Input: part model. Units: mm. Frame: model coordinates. A direction names the side the tool comes from. Coordinates: 2 decimals unless noted, no trailing zeros. Write each loop counter-clockwise with the first axis right and the second up, starting at its lowest first coordinate (ties: lowest second). Pieces come first, ordered by that corner, then holes. Notation, with made-up numbers: (-10, 7.5) - (1, 7.5) arc R13 ccw to (1, 23.5) - close; hole circle Ø2 at (-2, 60). An arc over 180 degrees is marked (long way). Use a Markdown table: item, result. Add a question column.
Q1. Pin query (flat end, axial travel): P1, Ø10, axis at x = -28.5, y = -15, coming from the -Z side; P2, Ø4, axis at x = -10.49, y = -152.4, coming from the -Z side; P3, Ø1.5, axis at x = -28.5, y = 143.5, coming from the -Z side; P4, Ø8.5, axis at y = -76.2, z = 228.6, coming from the +X side. Return the tip coordinate at first contact, or that it passes through.
Q2. Set-up query: faces 1 (the face through (1.6, 3, 3)), 2 (the face through (-36, -3, -217.5)), 3 (the face through (-35, -3, -215.9)), 4 (the face through (-12, -3, 242.9)), 5 (the face through (-23.8, -3, 226)). Return all of +Z, -Z, +X, -X, +Y, -Y with unobstructed straight access to the full face (end or side cutting, diameter ignored); none if empty.
Q3. Section query A-A (y = -59). Return the cut outline in (x, z).
Q4. Mould query, pull axis Z, two halves, no side actions, for faces 6 (the face through (1, -190.5, -73)), 7 (the face through (-23.513, 3, -229)), 8 (the face through (-12, -3, 241.3)), 9 (the face through (-14, 3, -242.9)). Classes: released by +Z, released by -Z, zero draft, split by the parting line, or undercut.
Q5. Section query B-B (z = -13). Return the cut outline in (x, y), then the cut area to 3 significant figures.
Q6. Material intervals for probe 1 along Y at (x, z) = (-24, 228); probe 2 along Z at (x, y) = (-7.5, 20); probe 3 along Y at (x, z) = (0.8, 228.6), sorted ascending. Write a range as from..to.
from build123d import *

# Parameters (mm, degrees)
SKETCH1_W                    = 482.6
SKETCH1_H                    = 381
BOSS_EXTRUDE1_DEPTH          = 1.6002
EDGE_FLANGE1_STRIP_W         = 9.6012
EDGE_FLANGE1_STRIP_H         = 1.6002
EDGE_FLANGE1_STRIP_CUT_DEPTH = 381
EDGE_FLANGE1_DEPTH           = 381
EDGE_FLANGE2_STRIP_W         = 9.6012
EDGE_FLANGE2_STRIP_H         = 1.6002
EDGE_FLANGE2_STRIP_CUT_DEPTH = 381
EDGE_FLANGE2_DEPTH           = 381
EDGE_FLANGE3_STRIP_W         = 9.6012
EDGE_FLANGE3_STRIP_H         = 1.6002
EDGE_FLANGE3_STRIP_CUT_DEPTH = 381
EDGE_FLANGE3_DEPTH           = 381
EDGE_FLANGE4_STRIP_W         = 9.6012
EDGE_FLANGE4_STRIP_H         = 1.6002
EDGE_FLANGE4_STRIP_CUT_DEPTH = 381
EDGE_FLANGE4_DEPTH           = 381
EDGE_FLANGE5_STRIP_W         = 9.6012
EDGE_FLANGE5_STRIP_H         = 1.6002
EDGE_FLANGE5_STRIP_CUT_DEPTH = 381
EDGE_FLANGE5_DEPTH           = 381
SKETCH24_R                   = 3.2639
CUT_EXTRUDE2_DEPTH           = 2.54
SKETCH25_R                   = 3.2639
CUT_EXTRUDE3_DEPTH           = 310.870566463
SKETCH26_R                   = 3.2639
CUT_EXTRUDE4_DEPTH           = 2.54
SKETCH27_R                   = 3.2639
CUT_EXTRUDE6_DEPTH           = 2.54
SKETCH29_R                   = 3.2639
CUT_EXTRUDE7_DEPTH           = 2.54


# Sheet-metal steps are written as plain solids
with BuildPart() as part:
    # Sketch1 → Boss-Extrude1 (new body)
    with BuildSketch(Plane(origin=(0, 0, 0), x_dir=(0, 0, -1), z_dir=(1, 0, 0))):
        Rectangle(SKETCH1_W, SKETCH1_H)
    extrude(amount=BOSS_EXTRUDE1_DEPTH)

    # Edge-Flange1 strip (across the edge) → Edge-Flange1 strip cut (cut)
    with BuildSketch(Plane(origin=(0, 190.5, -241.3), x_dir=(0, 0, 1), z_dir=(0, -1, 0))):
        with Locations((-3.2004, -0.8001)):
            Rectangle(EDGE_FLANGE1_STRIP_W, EDGE_FLANGE1_STRIP_H)
    extrude(amount=EDGE_FLANGE1_STRIP_CUT_DEPTH, mode=Mode.SUBTRACT)

    # Edge-Flange1 section (across the edge) → Edge-Flange1 (add)
    with BuildSketch(Plane(origin=(0, 190.5, -241.3), x_dir=(0, 0, 1), z_dir=(0, -1, 0))):
        with BuildLine():
            Line((-1.6002, 1.6002), (-1.6002, 23.51278))
            Line((-1.6002, 23.51278), (0, 23.51278))
            Line((0, 23.51278), (0, 1.6002))
            ThreePointArc((0, 1.6002), (0.468687729, 0.468687729), (1.6002, 0))
            Line((1.6002, 0), (1.6002, -1.6002))
            ThreePointArc((1.6002, -1.6002), (-0.662824543, -0.662824543), (-1.6002, 1.6002))
        make_face()
    extrude(amount=EDGE_FLANGE1_DEPTH)

    # Edge-Flange2 strip (across the edge) → Edge-Flange2 strip cut (cut)
    with BuildSketch(Plane(origin=(-23.51278, 190.5, -241.3), x_dir=(1, 0, 0), z_dir=(0, -1, 0))):
        with Locations((-3.2004, -0.8001)):
            Rectangle(EDGE_FLANGE2_STRIP_W, EDGE_FLANGE2_STRIP_H)
    extrude(amount=EDGE_FLANGE2_STRIP_CUT_DEPTH, mode=Mode.SUBTRACT)

    # Edge-Flange2 section (across the edge) → Edge-Flange2 (add)
    with BuildSketch(Plane(origin=(-23.51278, 190.5, -241.3), x_dir=(1, 0, 0), z_dir=(0, -1, 0))):
        with BuildLine():
            Line((-1.6002, 1.6002), (-1.6002, 23.7998))
            Line((-1.6002, 23.7998), (0, 23.7998))
            Line((0, 23.7998), (0, 1.6002))
            ThreePointArc((0, 1.6002), (0.468687729, 0.468687729), (1.6002, 0))
            Line((1.6002, 0), (1.6002, -1.6002))
            ThreePointArc((1.6002, -1.6002), (-0.662824543, -0.662824543), (-1.6002, 1.6002))
        make_face()
    extrude(amount=EDGE_FLANGE2_DEPTH)

    # Edge-Flange3 strip (across the edge) → Edge-Flange3 strip cut (cut)
    with BuildSketch(Plane(origin=(-25.11298, -190.5, -217.5002), x_dir=(0, 0, -1), z_dir=(0, 1, 0))):
        with Locations((-3.2004, -0.8001)):
            Rectangle(EDGE_FLANGE3_STRIP_W, EDGE_FLANGE3_STRIP_H)
    extrude(amount=EDGE_FLANGE3_STRIP_CUT_DEPTH, mode=Mode.SUBTRACT)

    # Edge-Flange3 section (across the edge) → Edge-Flange3 (add)
    with BuildSketch(Plane(origin=(-25.11298, -190.5, -217.5002), x_dir=(0, 0, -1), z_dir=(0, 1, 0))):
        with BuildLine():
            Line((-1.6002, 1.6002), (-1.6002, 23.7998))
            Line((-1.6002, 23.7998), (0, 23.7998))
            Line((0, 23.7998), (0, 1.6002))
            ThreePointArc((0, 1.6002), (0.468687729, 0.468687729), (1.6002, 0))
            Line((1.6002, 0), (1.6002, -1.6002))
            ThreePointArc((1.6002, -1.6002), (-0.662824543, -0.662824543), (-1.6002, 1.6002))
        make_face()
    extrude(amount=EDGE_FLANGE3_DEPTH)

    # Edge-Flange4 strip (across the edge) → Edge-Flange4 strip cut (cut)
    with BuildSketch(Plane(origin=(0, -190.5, 241.3), x_dir=(0, 0, -1), z_dir=(0, 1, 0))):
        with Locations((-3.2004, -0.8001)):
            Rectangle(EDGE_FLANGE4_STRIP_W, EDGE_FLANGE4_STRIP_H)
    extrude(amount=EDGE_FLANGE4_STRIP_CUT_DEPTH, mode=Mode.SUBTRACT)

    # Edge-Flange4 section (across the edge) → Edge-Flange4 (add)
    with BuildSketch(Plane(origin=(0, -190.5, 241.3), x_dir=(0, 0, -1), z_dir=(0, 1, 0))):
        with BuildLine():
            Line((-1.6002, 1.6002), (-1.6002, 23.7998))
            Line((-1.6002, 23.7998), (0, 23.7998))
            Line((0, 23.7998), (0, 1.6002))
            ThreePointArc((0, 1.6002), (0.468687729, 0.468687729), (1.6002, 0))
            Line((1.6002, 0), (1.6002, -1.6002))
            ThreePointArc((1.6002, -1.6002), (-0.662824543, -0.662824543), (-1.6002, 1.6002))
        make_face()
    extrude(amount=EDGE_FLANGE4_DEPTH)

    # Edge-Flange5 strip (across the edge) → Edge-Flange5 strip cut (cut)
    with BuildSketch(Plane(origin=(-23.7998, -190.5, 241.3), x_dir=(1, 0, 0), z_dir=(0, 1, 0))):
        with Locations((-3.2004, -0.8001)):
            Rectangle(EDGE_FLANGE5_STRIP_W, EDGE_FLANGE5_STRIP_H)
    extrude(amount=EDGE_FLANGE5_STRIP_CUT_DEPTH, mode=Mode.SUBTRACT)

    # Edge-Flange5 section (across the edge) → Edge-Flange5 (add)
    with BuildSketch(Plane(origin=(-23.7998, -190.5, 241.3), x_dir=(1, 0, 0), z_dir=(0, 1, 0))):
        with BuildLine():
            Line((-1.6002, 1.6002), (-1.6002, 23.7998))
            Line((-1.6002, 23.7998), (0, 23.7998))
            Line((0, 23.7998), (0, 1.6002))
            ThreePointArc((0, 1.6002), (0.468687729, 0.468687729), (1.6002, 0))
            Line((1.6002, 0), (1.6002, -1.6002))
            ThreePointArc((1.6002, -1.6002), (-0.662824543, -0.662824543), (-1.6002, 1.6002))
        make_face()
    extrude(amount=EDGE_FLANGE5_DEPTH)

    # Sketch24 → Cut-Extrude2 (cut)
    with BuildSketch(Plane.XY.offset(-215.9)):
        with Locations((-38.04158, 152.4)):
            Circle(SKETCH24_R)
        with Locations((-38.04158, 76.2)):
            Circle(SKETCH24_R)
        with Locations((-38.04158, 0)):
            Circle(SKETCH24_R)
        with Locations((-38.04158, -76.2)):
            Circle(SKETCH24_R)
        with Locations((-38.04158, -152.4)):
            Circle(SKETCH24_R)
    extrude(amount=-CUT_EXTRUDE2_DEPTH, mode=Mode.SUBTRACT)

    # Sketch25 → Cut-Extrude3 (cut, through all)
    with BuildSketch(Plane.ZY.offset(25.4)):
        with Locations((228.6, 152.4)):
            Circle(SKETCH25_R)
        with Locations((228.6, 76.2)):
            Circle(SKETCH25_R)
        with Locations((228.6, -76.2)):
            Circle(SKETCH25_R)
        with Locations((228.6, -152.4)):
            Circle(SKETCH25_R)
        with Locations((228.6, 0)):
            Circle(SKETCH25_R)
    extrude(amount=-CUT_EXTRUDE3_DEPTH, mode=Mode.SUBTRACT)

    # Sketch26 → Cut-Extrude4 (cut)
    with BuildSketch(Plane(origin=(0, 0, -242.9002), x_dir=(-1, 0, 0), z_dir=(0, 0, -1))):
        with Locations((10.4902, 152.4)):
            Circle(SKETCH26_R)
        with Locations((10.4902, 76.2)):
            Circle(SKETCH26_R)
        with Locations((10.4902, 0)):
            Circle(SKETCH26_R)
        with Locations((10.4902, -76.2)):
            Circle(SKETCH26_R)
        with Locations((10.4902, -152.4)):
            Circle(SKETCH26_R)
    extrude(amount=-CUT_EXTRUDE4_DEPTH, mode=Mode.SUBTRACT)

    # Sketch27 → Cut-Extrude6 (cut)
    with BuildSketch(Plane(origin=(1.6002, 0, 0), x_dir=(0, 0, -1), z_dir=(1, 0, 0))):
        with Locations((-214.2998, 178.689)):
            Circle(SKETCH27_R)
        with Locations((-106.3498, 178.689)):
            Circle(SKETCH27_R)
        with Locations((1.6002, 178.689)):
            Circle(SKETCH27_R)
        with Locations((109.5502, 178.689)):
            Circle(SKETCH27_R)
        with Locations((217.5002, 178.689)):
            Circle(SKETCH27_R)
    extrude(amount=-CUT_EXTRUDE6_DEPTH, mode=Mode.SUBTRACT)

    # Sketch29 → Cut-Extrude7 (cut)
    with BuildSketch(Plane.ZY):
        with Locations((-192.1002, -178.7144)):
            Circle(SKETCH29_R)
        with Locations((-90.5002, -178.7144)):
            Circle(SKETCH29_R)
        with Locations((11.0998, -178.7144)):
            Circle(SKETCH29_R)
        with Locations((112.6998, -178.7144)):
            Circle(SKETCH29_R)
        with Locations((214.2998, -178.7144)):
            Circle(SKETCH29_R)
    extrude(amount=-CUT_EXTRUDE7_DEPTH, mode=Mode.SUBTRACT)


solid = part.part
Values follow:
| question | item | result |
|---|---|---|
| 1 | P1 | z = -242.48 |
| 1 | P2 | z = 241.3 |
| 1 | P3 | z = -217.5 |
| 1 | P4 | x = 1.6 |
| 2 | face 1 | +Z, -Z, +X, +Y, -Y |
| 2 | face 2 | -Z, -X, +Y, -Y |
| 2 | face 3 | +Z, -X, +Y, -Y |
| 2 | face 4 | +Z, +X, -X, +Y, -Y |
| 2 | face 5 | +Y, -Y |
| 3 | outline | (-48.91, -217.5) - (-26.71, -217.5) arc R1.6 cw to (-25.11, -219.1) - (-25.11, -239.7) arc R3.2 ccw to (-21.91, -242.9) - (-1.6, -242.9) arc R3.2 ccw to (1.6, -239.7) - (1.6, 239.7) arc R3.2 ccw to (-1.6, 242.9) - (-22.2, 242.9) arc R3.2 ccw to (-25.4, 239.7) - (-25.4, 217.5) - (-23.8, 217.5) - (-23.8, 239.7) arc R1.6 cw to (-22.2, 241.3) - (-1.6, 241.3) arc R1.6 cw to (0, 239.7) - (0, -239.7) arc R1.6 cw to (-1.6, -241.3) - (-21.91, -241.3) arc R1.6 cw to (-23.51, -239.7) - (-23.51, -219.1) arc R3.2 ccw to (-26.71, -215.9) - (-48.91, -215.9) - close |
| 4 | face 6 | zero draft |
| 4 | face 7 | undercut |
| 4 | face 8 | undercut |
| 4 | face 9 | released by -Z |
| 5 | outline | (0, -190.5) - (1.6, -190.5) - (1.6, 190.5) - (0, 190.5) - close |
| 5 | area | 610 mm2 |
| 6 | probe 1 | -190.5..-155.61, -149.19..-79.41, -72.99..-3.21, 3.21..72.99, 79.41..149.19, 155.61..190.5 |
| 6 | probe 2 | -242.9..-241.3, 241.3..242.9 |
| 6 | probe 3 | -190.5..-155.66, -149.14..-79.46, -72.94..-3.26, 3.26..72.94, 79.46..149.14, 155.66..190.5 |
